Model file for the job. Use its own axes, mm. Round coordinates to 2 decimals unless told otherwise and drop trailing zeros. Order: outer loops, then holes, each group sorted by start corner. A loop starts at its lowest first (then second) coordinate and runs counter-clockwise, first axis right, second up. Notation, with made-up numbers: (24.25, -35) -> (82.25, -35) arc R5 cw to (82.25, -31) -> close; hole circle Ø9 at (49, 57). An arc over 180 degrees is marked (long way). Use CSV: the item, a comma, the result in double quotes.
```python
from build123d import *

# Parameters (mm, degrees)
BOSS_EXTRUDE1_DEPTH = 5
SKETCH3_R           = 1.475
CUT_EXTRUDE1_DEPTH  = 137.064643721
SKETCH4_R           = 22.5
SKETCH4_R_2         = 1.975
SKETCH4_R_3         = 1.4
SKETCH4_R_4         = 1.475
CUT_EXTRUDE2_DEPTH  = 137.064643721


with BuildPart() as part:
    # Sketch2 → Boss-Extrude1 (new body)
    with BuildSketch(Plane(origin=(0, 0, 0), x_dir=(1, 0, 0), z_dir=(0, 1, 0))):
        with BuildLine():
            Line((-52.202038886, 61.082677165), (85.797961114, 61.082677165))
            ThreePointArc((85.797961114, 61.082677165), (90.6611457, 59.421487905), (92.797961114, 54.747717054))
            Line((92.797961114, 54.747717054), (92.797961114, -62.252282946))
            ThreePointArc((92.797961114, -62.252282946), (90.782438223, -67.143884297), (85.797961114, -68.917322835))
            Line((85.797961114, -68.917322835), (-52.202038886, -68.917322835))
            ThreePointArc((-52.202038886, -68.917322835), (-117.202038886, -3.917322835), (-52.202038886, 61.082677165))
        make_face()
    extrude(amount=BOSS_EXTRUDE1_DEPTH)

    # Sketch3 → Cut-Extrude1 (cut, through all)
    with BuildSketch(Plane(origin=(0, 5, 0), x_dir=(1, 0, 0), z_dir=(0, 1, 0))):
        with Locations(Location((86.297961114, 54.582677165, 0), (0, 0, 270))):
            Circle(SKETCH3_R)
        with Locations(Location((-52.202038886, 54.582677165, 0), (0, 0, 270))):
            Circle(SKETCH3_R)
        with Locations(Location((-110.702038886, -3.912214457, 0), (0, 0, 270))):
            Circle(SKETCH3_R)
        with Locations(Location((86.297961114, -62.417322835, 0), (0, 0, 90))):
            Circle(SKETCH3_R)
        with Locations(Location((-52.110168441, -62.417322835, 0), (0, 0, 90))):
            Circle(SKETCH3_R)
    extrude(amount=-CUT_EXTRUDE1_DEPTH, mode=Mode.SUBTRACT)

    # Sketch4 → Cut-Extrude2 (cut, through all)
    with BuildSketch(Plane(origin=(0, 5, 0), x_dir=(1, 0, 0), z_dir=(0, 1, 0))):
        with Locations(Location((-52.202038886, -3.822023973, 0), (0, 0, 270))):
            Circle(SKETCH4_R)
        with Locations(Location((-72.538754153, 16.367031882, 0), (0, 0, 270))):
            Circle(SKETCH4_R_2)
        with Locations(Location((31.047961114, 14.627976027, 0), (0, 0, 270))):
            Circle(SKETCH4_R_3)
        with Locations(Location((35.409642143, 27.67666392, 0), (0, 0, 270))):
            Circle(SKETCH4_R_4)
        with Locations(Location((84.87537154, 27.67666392, 0), (0, 0, 90))):
            Circle(SKETCH4_R_4)
        with Locations(Location((84.87537154, -36.84883921, 0), (0, 0, 270))):
            Circle(SKETCH4_R_4)
        with Locations(Location((35.409642143, -36.84883921, 0), (0, 0, 90))):
            Circle(SKETCH4_R_4)
        with Locations(Location((-72.538388848, -24.642968116, 0), (0, 0, 270))):
            Circle(SKETCH4_R_2)
        with Locations(Location((-31.529119459, -24.642968116, 0), (0, 0, 90))):
            Circle(SKETCH4_R_2)
        with Locations(Location((-31.528754153, 16.367031882, 0), (0, 0, 90))):
            Circle(SKETCH4_R_2)
        Polygon((37.938439462, 15.24849763), (37.938439462, -20.06020818), (40.938439462, -24.262255151), (78.657482766, -24.262255151), (81.772324977, -20.06020818), (81.542640555, 15.24849763), (78.657482766, 18.237744849), (40.938439462, 18.237744849), align=None)
        with BuildLine():
            Line((17.447961114, 16.027976027), (14.647961114, 16.027976027))
            ThreePointArc((14.647961114, 16.027976027), (13.689795357, 14.627976027), (14.647961114, 13.227976027))
            Line((14.647961114, 13.227976027), (17.447961114, 13.227976027))
            ThreePointArc((17.447961114, 13.227976027), (18.651293074, 14.627976027), (17.447961114, 16.027976027))
        make_face()
    extrude(amount=-CUT_EXTRUDE2_DEPTH, mode=Mode.SUBTRACT)


solid = part.part
```
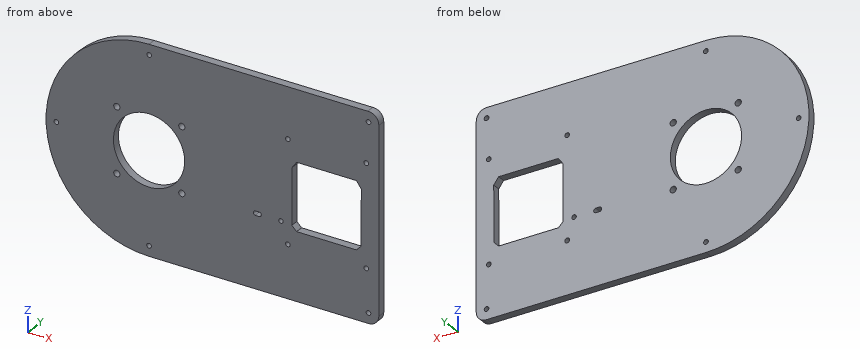
Q1. Cut at B-B (y = 1.6). State how many separate pieces and enclosed holes the cut face has, plus the area to 3 significant figures.
From the geometry:
separate pieces,"1"
enclosed holes,"17"
area,"21,900 mm²"
Q2. Cut at C-C (z = 33). Give the cut face in (x, y).
From the geometry:
outline,"(-110.33, 0) -> (92.8, 0) -> (92.8, 5) -> (-110.33, 5) -> close"
Q3. Probe line 1 along Z through (x, y) = (73, 0.8); line 2 along X through (y, z) = (2.15, 9); line 3 along X through (y, z) = (1.35, 13.5). List the from-to ranges inside material, lowest first.
From the geometry:
line 1,"z = -61.08 to -18.24, 24.26 to 68.92"
line 2,"x = -117 to -74.1, -30.31 to 37.94, 81.7 to 92.8"
line 3,"x = -116.49 to -72.51, -31.89 to 37.94, 81.73 to 92.8"
Q4. Cut at A-A (z = 8.5). Give the cut face in (x, y).
From the geometry:
outline,"(-117.04, 0) -> (-74.21, 0) -> (-74.21, 5) -> (-117.04, 5) -> close; (-30.19, 0) -> (37.94, 0) -> (37.94, 5) -> (-30.19, 5) -> close; (81.7, 0) -> (92.8, 0) -> (92.8, 5) -> (81.7, 5) -> close"
Q5. Pin check, flat tips, straight feed: pin 1 (2.5 mm diameter, centred on x = 35.41, z = 36.85, fed in from +Y); pin 2 (1.5 mm diameter, centred on y = 1.5, z = 24.5, fed in from +X); pin 3 (2.5 mm diameter, centred on x = 25.5, y = 2, fed in from -Z); pin 4 (0.8 mm diameter, centred on x = 15.5, y = 1.5, fed in from +Z). Stop position of each tip, or through.
From the geometry:
pin 1,"passes through"
pin 2,"stops at x = 92.8"
pin 3,"stops at z = -61.08"
pin 4,"stops at z = 68.92"
Q6. Cut at D-D (x = -85.5). Give the cut face in (y, z).
From the geometry:
outline,"(0, -51.91) -> (5, -51.91) -> (5, 59.74) -> (0, 59.74) -> close"
